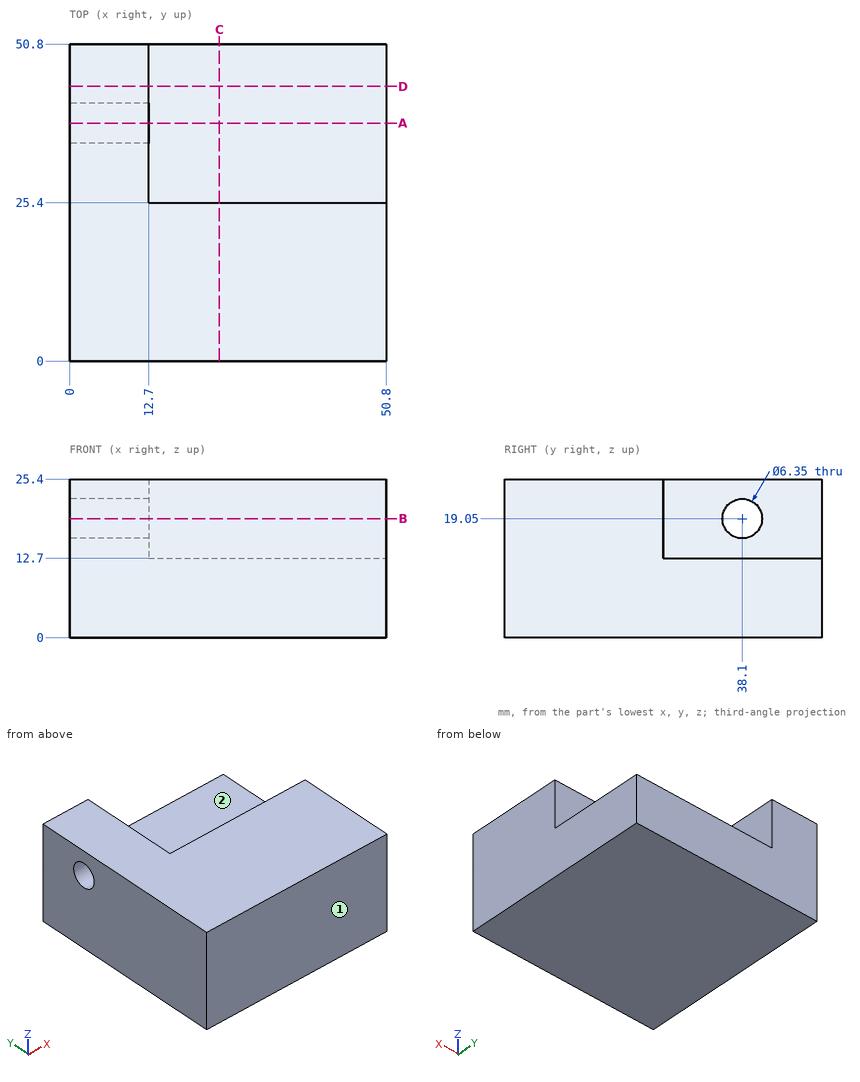
Verification items for this drawing (mm, ordinates from the low corner). A direction names the side the tool comes from. Round coordinates to 2 decimals unless told otherwise and drop trailing zeros. Loops run counter-clockwise (first coordinate to the right, second up) from the corner with the lowest first, then second, coordinate; pieces in that order, holes last. Notation, with made-up numbers: M -8.5,7.5 L 11.5,7.5 A24 cw 11.5,27.5 Z; hole C 34,17 d3. An arc over 180 degrees is marked long. Answer as a JSON object with one key per item and string values.
1. Section check D-D (y = 44). Record the boundary of the cut face in (x, z).
Reply:
{"outline": "M 0,0 L 50.8,0 L 50.8,12.7 L 12.7,12.7 L 12.7,25.4 L 0,25.4 Z"}
2. Gauge pin test, flat ends, axial feed: P1, Ø1, axis at y = 32.5, z = 16.5, coming from the +X side; P2, Ø2, axis at x = 14, y = 30, coming from the +Z side. Record the tip position at first contact, or that the pin passes through.
Reply:
{"P1": "stops at x = 12.7", "P2": "stops at z = 12.7"}
3. Section check A-A (y = 38.1). Record the boundary of the cut face in (x, z) (3 decimals), plus the area to 3 significant figures.
Reply:
{"outline": "M 0,0 L 50.8,0 L 50.8,12.7 L 12.7,12.7 L 12.7,15.875 L 0,15.875 Z; M 0,22.225 L 12.7,22.225 L 12.7,25.4 L 0,25.4 Z", "area": "726 mm²"}
4. Section check C-C (x = 24). Record the boundary of the cut face in (y, z), plus the area to 3 significant figures.
Reply:
{"outline": "M 0,0 L 50.8,0 L 50.8,12.7 L 25.4,12.7 L 25.4,25.4 L 0,25.4 Z", "area": "968 mm²"}
5. Scan lines: line 1 (Z direction, x = 8.5, y = 38.1) (3 decimals); line 2 (X direction, y = 43, z = 17.75); line 3 (Z direction, x = 11, y = 40). Record each from-to range of solid material in increasing order.
Reply:
{"line 1": "z = 0 to 15.875, 22.225 to 25.4", "line 2": "x = 0 to 12.7", "line 3": "z = 0 to 16.51, 21.59 to 25.4"}
6. Section check B-B (z = 19.05). Record the boundary of the cut face in (x, y) (3 decimals), plus the area to 3 significant figures.
Reply:
{"outline": "M 0,0 L 50.8,0 L 50.8,25.4 L 12.7,25.4 L 12.7,34.925 L 0,34.925 Z; M 0,41.275 L 12.7,41.275 L 12.7,50.8 L 0,50.8 Z", "area": "1,530 mm²"}
7. Access from +Z, -Z, +X, -X, +Y, -Y to the whole of each face (thin tool, end or side, straight path). Record for the marked faces 1 and 2.
Reply:
{"face 1": "+Z, -Z, +X, -X, -Y", "face 2": "+Z, +X, +Y"}
